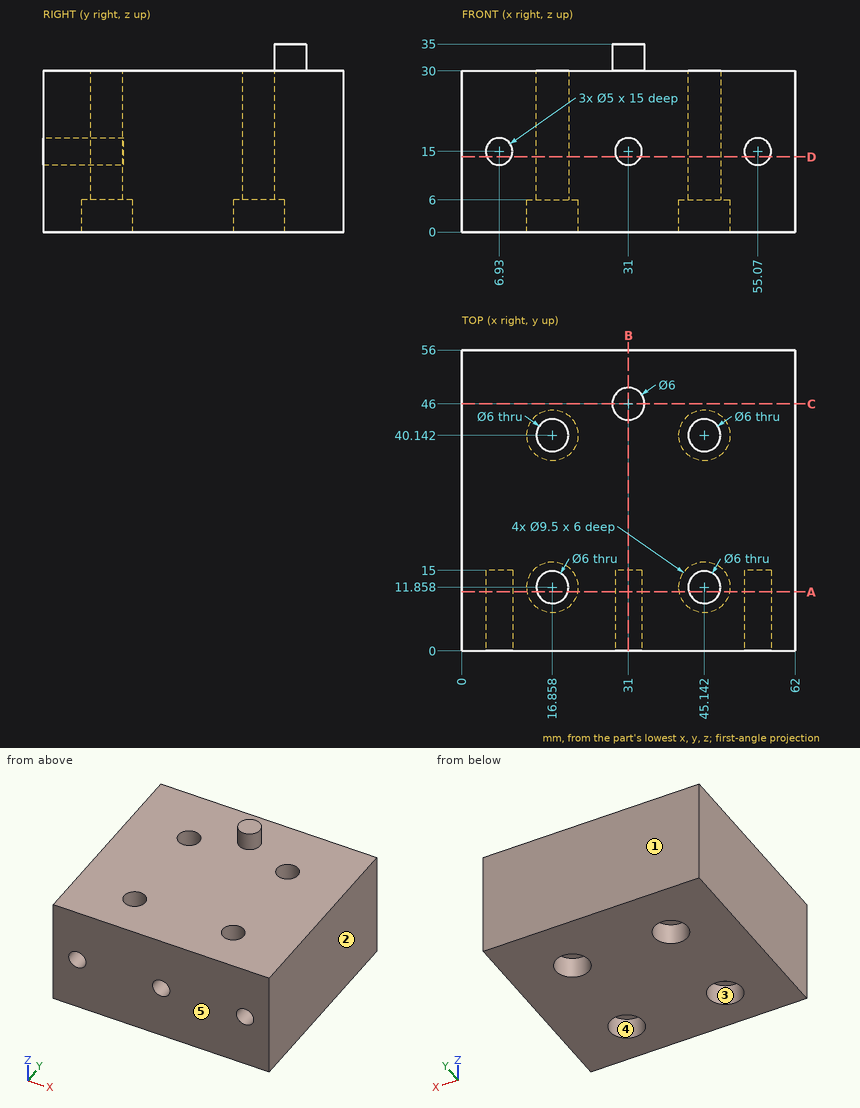
Here's the drawing with two shaded views (mm, measured from the low corner). I have some questions. A direction names the side the tool comes from. Give positions to 0.01 mm unless a question says otherwise; leave off trailing zeros. Loops run counter-clockwise (first coordinate to the right, second up) from the corner with the lowest first, then second, coordinate; pieces in that order, holes last. Notation, with made-up numbers: (43.25, -1) - (50.25, -1) arc R28 cw to (50.25, 34) - close; hole circle Ø9 at (53.5, 2). An arc over 180 degrees is marked (long way). Answer in a Markdown table with one row per item. Add a question column.
Q1. If we section it at C-C (y = 46): List the corners of the cut face in (x, z) for me, plus the area to 3 significant figures.
Q2. If we section it at A-A (y = 11): List the corners of the cut face in (x, z) for me, plus the area to 3 significant figures.
Q3. Please list where these lines run through material, in increasing order: L1, parallel to X at y = 40, z = 19; L2, parallel to Y at x = 49.5, z = 5; L3, parallel to X at y = 9.5, z = 15. Write a range as from..to.
Q4. Which directions (+Z, -Z, +X, -X, +Y, -Y) give clear straight access to the entire face, cutting with the end or side of a thin tool? Please do the marked faces 4 and 5.
Q5. We'd pull the mould along Y, two halves only. Please class the marked faces 1, 2 and 3: +Y half, -Y half, draft (parallel to the pull), parting line (faces both ways), or undercut.
Q6. For pin 1 (3 mm diameter, centred on x = 15, y = 38, fed in from -Z); pin 2 (8.5 mm diameter, centred on x = 45.14, y = 40.14, fed in from +Z), each with a flat end and sliding along its axis, tell me the tip position at first contact or that it passes through.
Q7. If we section it at B-B (x = 31): List the corners of the cut face in (y, z) for me.
Q8. If we section it at D-D (z = 14): List the corners of the cut face in (x, y) for me.
The answers:
| question | item | result |
|---|---|---|
| 1 | outline | (0, 0) - (62, 0) - (62, 30) - (34, 30) - (34, 35) - (28, 35) - (28, 30) - (0, 30) - close |
| 1 | area | 1,890 mm^2 |
| 2 | outline | (0, 0) - (12.19, 0) - (12.19, 6) - (13.98, 6) - (13.98, 30) - (0, 30) - close; (19.73, 6) - (21.53, 6) - (21.53, 0) - (40.47, 0) - (40.47, 6) - (42.27, 6) - (42.27, 30) - (19.73, 30) - close; (48.02, 6) - (49.81, 6) - (49.81, 0) - (62, 0) - (62, 30) - (48.02, 30) - close; hole circle Ø5 at (6.93, 15); hole circle Ø5 at (31, 15); hole circle Ø5 at (55.07, 15) |
| 2 | area | 1,410 mm^2 |
| 3 | L1 | x = 0..13.86, 19.85..42.15, 48.14..62 |
| 3 | L2 | y = 0..9.97, 13.75..38.25, 42.03..56 |
| 3 | L3 | x = 0..4.43, 9.43..15, 18.71..28.5, 33.5..43.29, 47..52.57, 57.57..62 |
| 4 | face 4 | -Z |
| 4 | face 5 | +Z, -Z, +X, -X, -Y |
| 5 | face 1 | +Y half |
| 5 | face 2 | draft |
| 5 | face 3 | undercut |
| 6 | pin 1 | stops at z = 6 |
| 6 | pin 2 | stops at z = 30 |
| 7 | outline | (0, 0) - (56, 0) - (56, 30) - (49, 30) - (49, 35) - (43, 35) - (43, 30) - (0, 30) - (0, 17.5) - (15, 17.5) - (15, 12.5) - (0, 12.5) - close |
| 8 | outline | (0, 0) - (4.64, 0) - (4.64, 15) - (9.22, 15) - (9.22, 0) - (28.71, 0) - (28.71, 15) - (33.29, 15) - (33.29, 0) - (52.78, 0) - (52.78, 15) - (57.36, 15) - (57.36, 0) - (62, 0) - (62, 56) - (0, 56) - close; hole circle Ø6 at (16.86, 11.86); hole circle Ø6 at (16.86, 40.14); hole circle Ø6 at (45.14, 11.86); hole circle Ø6 at (45.14, 40.14) |
